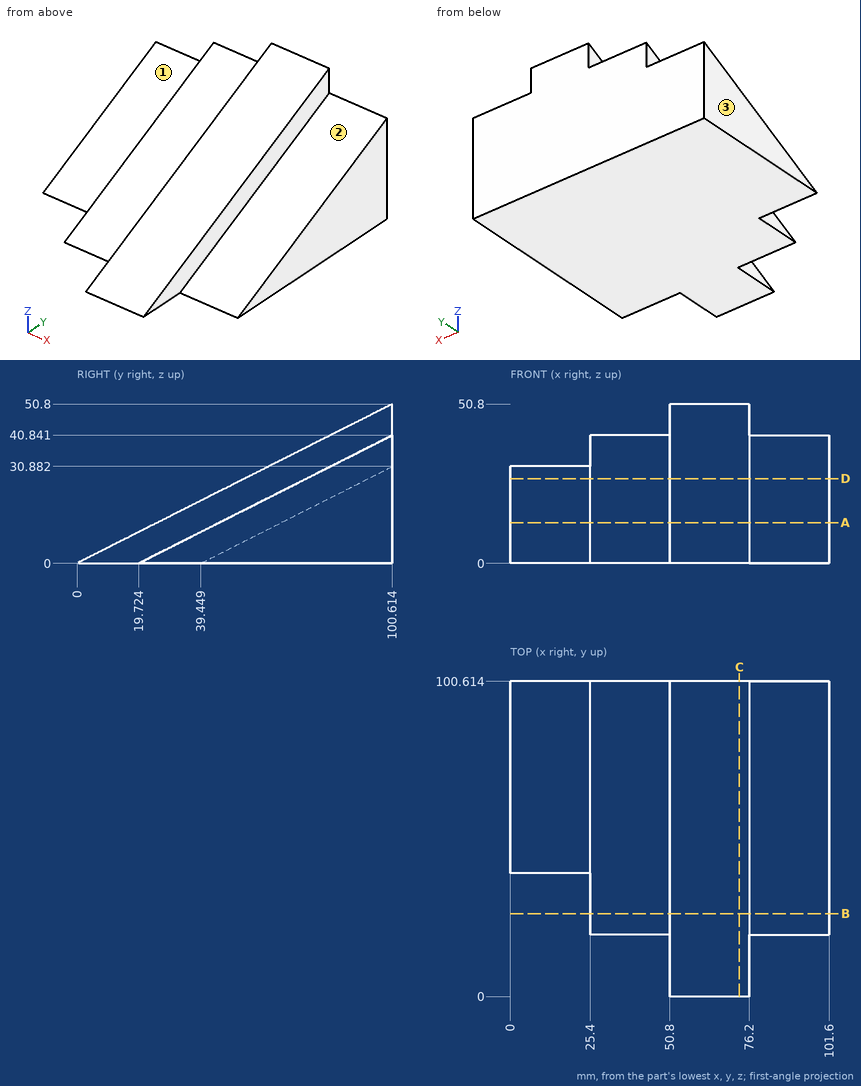
Part print with two shaded views. Sizes in mm from the minimum x, y, z corner. A direction names the side the tool comes from. Coordinates: 2 decimals unless noted, no trailing zeros. Order: outer loops, then holes, each group sorted by start corner. A loop starts at its lowest first (then second) coordinate and runs counter-clockwise, first axis right, second up. Notation, with made-up numbers: M -15,-38.75 L 34,-38.75 A29 cw 34,-14.75 Z; hole C 41.25,47.5 d4. An arc over 180 degrees is marked long. One line per question, with ' | ' between items. Start each with the question number.
1. Cut at D-D (z = 27). Write the cut outline in (x, y) (1 decimal).
2. Cut at A-A (z = 13). Write the cut outline in (x, y), plus the area to 3 significant figures.
3. Cut at C-C (x = 73). Write the cut outline in (y, z).
4. Wall check: line 1 along X through (y, z) = (59, 21.5); line 2 along X through (y, z) = (27.5, 3.5); line 3 along Z through (x, y) = (44, 25) (1 decimal). Give the ranges that are in metal, low to high. Write a range as [from, to].
5. Flat gauge pins, fed straight in: P1, Ø4, axis at y = 88.5, z = 40, coming from the +X side; P2, Ø10, axis at y = 63, z = 19.5, coming from the -X side; P3, Ø10, axis at y = 48.5, z = 8.5, coming from the -X side; P4, Ø5, axis at y = 30, z = 19, coming from the -X side (1 decimal). Where does each tip first touch, or does it go through?
6. Cut at B-B (y = 26.5). Write the cut outline in (x, z).
7. Tool access for the marked faces 1, 2 and 3: list every direction of +Z, -Z, +X, -X, +Y, -Y with a clear straight run to the whole face (end or side of a thin tool).
The answers:
1) outline: M 0,92.9 L 25.4,92.9 L 25.4,73.2 L 50.8,73.2 L 50.8,53.5 L 76.2,53.5 L 76.2,73.2 L 101.6,73.2 L 101.6,100.6 L 0,100.6 Z
2) outline: M 0,65.2 L 25.4,65.2 L 25.4,45.47 L 50.8,45.47 L 50.8,25.75 L 76.2,25.75 L 76.2,45.47 L 101.6,45.47 L 101.6,100.61 L 0,100.61 Z | area: 5,600 mm2
3) outline: M 0,0 L 100.61,0 L 100.61,50.8 Z
4) line 1: x = [50.8, 76.2] | line 2: x = [25.4, 101.6] | line 3: z = [0, 2.7]
5) P1: stops at x = 76.2 | P2: stops at x = 25.4 | P3: stops at x = 0 | P4: passes through
6) outline: M 25.4,0 L 101.6,0 L 101.6,3.42 L 76.2,3.42 L 76.2,13.38 L 50.8,13.38 L 50.8,3.42 L 25.4,3.42 Z
7) face 1: +Z, -X, -Y | face 2: +Z, +X, -Y | face 3: +Z, -Z, -X, +Y, -Y
